The listing builds one solid part. Answer for the finished solid, in the listing's coordinates (mm). Face numbers are marked on the shaded views. A direction names the side the tool comes from. Give positions to 0.01 mm unless a question says otherwise; leave off trailing zeros. Write each loop counter-clockwise with the first axis right and the second up, starting at its lowest first coordinate (ties: lowest second). Pieces come first, ordered by that corner, then holes. Notation, with made-up numbers: (30.5, 16) - (68.5, 16) arc R25 cw to (68.5, 30) - close; hole circle Ø3 at (8.25, 20). An arc over 180 degrees is marked (long way). Answer in a Markdown table with one row per item. Add a question column.
from build123d import *

# Parameters (mm, degrees)
SKETCH_1_W          = 40
SKETCH_1_H          = 42
SKETCH_1_R          = 1.55
EXTRUDE_1_DEPTH     = 3
SKETCH_2_W          = 40
SKETCH_2_H          = 3
EXTRUDE_2_DEPTH     = 49
SKETCH_3_R          = 11.5
SKETCH_3_R_2        = 1.55
CUT_EXTRUDE_1_DEPTH = 49
FILLET_1_R          = 5
FILLET_2_R          = 3


with BuildPart() as part:
    # 草图1 → 凸台-拉伸1 (new body)
    with BuildSketch(Plane(origin=(0, 0, 0), x_dir=(1, 0, 0), z_dir=(0, 1, 0))):
        Rectangle(SKETCH_1_W, SKETCH_1_H)
        with Locations(Location((-15, -12, 0), (0, 0, 270))):
            Circle(SKETCH_1_R, mode=Mode.SUBTRACT)
        with Locations(Location((-15, 12, 0), (0, 0, 270))):
            Circle(SKETCH_1_R, mode=Mode.SUBTRACT)
        with Locations(Location((15, 12, 0), (0, 0, 270))):
            Circle(SKETCH_1_R, mode=Mode.SUBTRACT)
        with Locations(Location((15, -12, 0), (0, 0, 270))):
            Circle(SKETCH_1_R, mode=Mode.SUBTRACT)
    extrude(amount=EXTRUDE_1_DEPTH)

    # 草图2 → 凸台-拉伸2 (add)
    with BuildSketch(Plane(origin=(0, 3, 0), x_dir=(1, 0, 0), z_dir=(0, 1, 0))):
        with Locations((0, 19.5)):
            Rectangle(SKETCH_2_W, SKETCH_2_H)
    extrude(amount=EXTRUDE_2_DEPTH)

    # 草图3 → 切除-拉伸1 (cut)
    with BuildSketch(Plane.XY.offset(-18)):
        with Locations((0, 31)):
            Circle(SKETCH_3_R)
        with Locations((-15.5, 46.5)):
            Circle(SKETCH_3_R_2)
        with Locations((15.5, 46.5)):
            Circle(SKETCH_3_R_2)
        with Locations((15.5, 15.5)):
            Circle(SKETCH_3_R_2)
        with Locations((-15.5, 15.5)):
            Circle(SKETCH_3_R_2)
    extrude(amount=-CUT_EXTRUDE_1_DEPTH, mode=Mode.SUBTRACT)

    # 圆角1
    fillet_1_edges = [part.edges().sort_by_distance(p)[0] for p in [
        (-20, 52, -19.5),
        (20, 52, -19.5),
        (20, 1.5, 21),
        (-20, 1.5, 21),
    ]]
    fillet(fillet_1_edges, radius=FILLET_1_R)

    # 圆角2
    fillet_2_edges = [part.edges().sort_by_distance(p)[0] for p in [
        (0, 3, -18),
    ]]
    fillet(fillet_2_edges, radius=FILLET_2_R)


solid = part.part
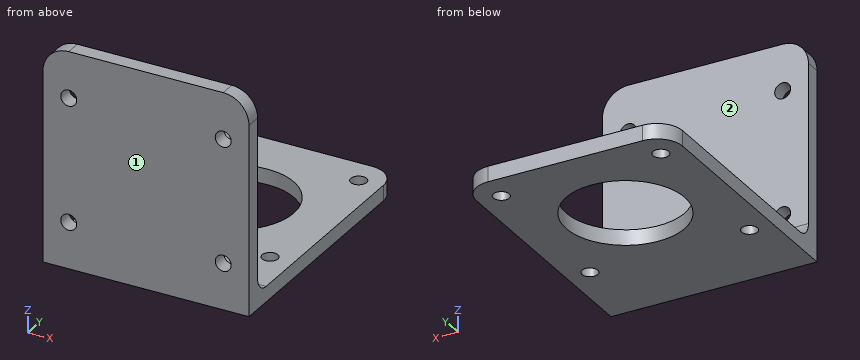
1. Section C-C (x = -9.5) is taken. Give the vertices of the cut face in (y, z), and give its area (3 significant figures).
2. Given pin 1 Ø12 at (x, y) = (-3.5, 45) entering from +Z; pin 2 Ø3.5 at (x, z) = (-15, 12) entering from +Y; pin 3 Ø5 at (x, y) = (0.5, 24.5) entering from -Z; pin 4 Ø5 at (x, y) = (-15.5, 15.5) entering from -Z, each flat-ended and moving along its own axis, determine where each tip first touches the part or whether it passes through.
3. Section B-B (z = -12) is taken. Give the vertices of the cut face in (x, y).
4. A tool of negligible diameter and unlimited length cuts with its end or side. For the marked faces 1 and 2, from which of +Z, -Z, +X, -X, +Y, -Y can it reach the whole face along a straight path? Write none if from no direction.
5. Section A-A (y = 31) is taken. Give the vertices of the cut face in (x, z).
6. Straight lines are drawn through the part: L1, parallel to X at y = 1.65, z = 12; L2, parallel to Y at x = 0.5, z = -19; L3, parallel to Y at x = 15, z = -20. For each, find the intervals that lie inside material, in ascending order. Write a range as [from, to].
7. Section D-D (y = 15.5) is taken. Give the vertices of the cut face in (x, z), and give its area (3 significant figures).
Geometry check:
| question | item | result |
|---|---|---|
| 1 | outline | (0, -21) - (24.52, -21) - (24.52, -18) - (6, -18) arc R3 cw to (3, -15) - (3, 21) - (0, 21) - close; (37.48, -21) - (52, -21) - (52, -18) - (37.48, -18) - close |
| 1 | area | 236 mm² |
| 2 | pin 1 | z = -18 |
| 2 | pin 2 | y = 3 |
| 2 | pin 3 | through |
| 2 | pin 4 | z = -21 |
| 3 | outline | (-20, 0) - (-16.55, 0) - (-16.55, 3) - (-20, 3) - close; (-13.45, 0) - (13.45, 0) - (13.45, 3) - (-13.45, 3) - close; (16.55, 0) - (20, 0) - (20, 3) - (16.55, 3) - close |
| 4 | face 1 | +Z, -Z, +X, -X, -Y |
| 4 | face 2 | +Z, +X, -X, +Y |
| 5 | outline | (-20, -21) - (-11.5, -21) - (-11.5, -18) - (-20, -18) - close; (11.5, -21) - (20, -21) - (20, -18) - (11.5, -18) - close |
| 6 | L1 | [-20, -16.55], [-13.45, 13.45], [16.55, 20] |
| 6 | L2 | [0, 19.51], [42.49, 52] |
| 6 | L3 | [0, 14.03], [16.97, 45.03], [47.97, 52] |
| 7 | outline | (-20, -21) - (-17.05, -21) - (-17.05, -18) - (-20, -18) - close; (-13.95, -21) - (13.95, -21) - (13.95, -18) - (-13.95, -18) - close; (17.05, -21) - (20, -21) - (20, -18) - (17.05, -18) - close |
| 7 | area | 101 mm² |
